from build123d import *

# Parameters (mm, degrees)
SKETCH1_R           = 2.1828125
BOSS_EXTRUDE1_DEPTH = 6.35
CHAMFER1_SIZE       = 0.396875


with BuildPart() as part:
    # Sketch1 → Boss-Extrude1 (new body)
    with BuildSketch(Plane(origin=(0, 0, 0), x_dir=(1, 0, 0), z_dir=(0, 1, 0))):
        with BuildLine():
            Line((-101.600254, 6.35), (0.000254, 6.35))
            ThreePointArc((0.000254, 6.35), (4.490202455, 4.490202455), (6.35, 0.000254))
            Line((6.35, 0.000254), (6.35, -12.700254))
            ThreePointArc((6.35, -12.700254), (4.490202455, -17.190202455), (0.000254, -19.05))
            ThreePointArc((0.000254, -19.05), (-4.490202455, -17.190202455), (-6.35, -12.700254))
            ThreePointArc((-6.35, -12.700254), (-8.209797545, -8.209797545), (-12.699746, -6.35))
            Line((-12.699746, -6.35), (-88.900254, -6.35))
            ThreePointArc((-88.900254, -6.35), (-93.390202455, -8.209797545), (-95.25, -12.699746))
            ThreePointArc((-95.25, -12.699746), (-97.109797545, -17.190202455), (-101.599746, -19.05))
            ThreePointArc((-101.599746, -19.05), (-106.090202455, -17.190202455), (-107.95, -12.700254))
            Line((-107.95, -12.700254), (-107.95, 0.000254))
            ThreePointArc((-107.95, 0.000254), (-106.090202455, 4.490202455), (-101.600254, 6.35))
        make_face()
        Circle(SKETCH1_R, mode=Mode.SUBTRACT)
        with Locations((-25.4, 0)):
            Circle(SKETCH1_R, mode=Mode.SUBTRACT)
        with Locations((-76.2, 0)):
            Circle(SKETCH1_R, mode=Mode.SUBTRACT)
        with Locations((-101.6, 0)):
            Circle(SKETCH1_R, mode=Mode.SUBTRACT)
        with Locations((-101.6, -12.7)):
            Circle(SKETCH1_R, mode=Mode.SUBTRACT)
        with Locations((0, -12.7)):
            Circle(SKETCH1_R, mode=Mode.SUBTRACT)
    extrude(amount=BOSS_EXTRUDE1_DEPTH)

    # Chamfer1
    chamfer1_edges = [part.edges().sort_by_distance(p)[0] for p in [
        (-4.490022844, 6.35, 17.19038206),
        (-50.8, 0, 6.35),
        (-93.390202455, 0, 8.209797545),
        (-97.10961794, 0, 17.190022844),
        (-4.490022844, 6.35, 17.19038206),
        (-97.10961794, 0, 17.190022844),
        (-106.090022844, 0, 17.19038206),
        (-106.090022844, 0, 17.19038206),
        (-107.95, 0, 6.35),
        (-106.090202455, 0, -4.490202455),
        (-50.8, 0, -6.35),
        (4.490202455, 0, -4.490202455),
        (6.35, 0, 6.35),
        (4.490202455, 0, 17.190202455),
        (-4.490022844, 0, 17.19038206),
        (4.490202455, 6.35, 17.190202455),
        (-4.490022844, 0, 17.19038206),
        (-8.20961794, 0, 8.209977156),
        (-8.20961794, 0, 8.209977156),
        (6.35, 6.35, 6.35),
        (4.490202455, 6.35, -4.490202455),
        (-50.8, 6.35, -6.35),
        (-106.090202455, 6.35, -4.490202455),
        (-2.1828125, 0, 0),
        (-2.1828125, 6.35, 0),
        (-107.95, 6.35, 6.35),
        (-27.5828125, 0, 0),
        (-27.5828125, 6.35, 0),
        (-106.090022844, 6.35, 17.19038206),
        (-78.3828125, 0, 0),
        (-78.3828125, 6.35, 0),
        (-106.090022844, 6.35, 17.19038206),
        (-8.20961794, 6.35, 8.209977156),
        (-103.7828125, 0, 0),
        (-103.7828125, 6.35, 0),
        (-97.10961794, 6.35, 17.190022844),
        (-103.7828125, 0, 12.7),
        (-103.7828125, 6.35, 12.7),
        (-97.10961794, 6.35, 17.190022844),
        (-2.1828125, 0, 12.7),
        (-2.1828125, 6.35, 12.7),
        (-93.390202455, 6.35, 8.209797545),
        (-50.8, 6.35, 6.35),
        (-8.20961794, 6.35, 8.209977156),
    ]]
    chamfer(chamfer1_edges, length=CHAMFER1_SIZE)


solid = part.part
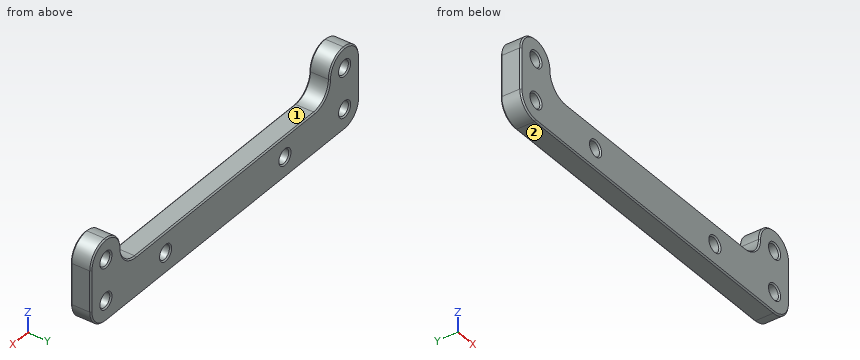
Part model, mm, in its own coordinate system. Face numbers are marked on the shaded views. A direction names the side the tool comes from. Coordinates: 2 decimals unless noted, no trailing zeros. Write each loop counter-clockwise with the first axis right and the second up, starting at its lowest first coordinate (ties: lowest second). Pieces come first, ordered by that corner, then holes. Notation, with made-up numbers: M 59.25,42 L 97.25,42 A29 cw 97.25,71 Z; hole C -13.5,69.5 d3. An arc over 180 degrees is marked long. Return JSON: item names as keys, results as strings.
1. Flat gauge pins, fed straight in: pin 1 Ø3 at (y, z) = (2.5, -3.5) entering from +X; pin 2 Ø5 at (x, z) = (-25.4, 0) entering from +Y; pin 3 Ø5 at (x, z) = (-93.5, 16) entering from +Y. Where does each tip first touch, or does it go through?
Determined:
{"pin 1": "x = 6.03", "pin 2": "y = 6.27", "pin 3": "y = 6.06"}
2. 3-axis set-ups, long thin cutter, end or side, ignore diameter. For the marked faces 1 and 2: which of +Z, -Z, +X, -X, +Y, -Y reach the whole face in a straight line?
Determined:
{"face 1": "+Z, +Y, -Y", "face 2": "-Z, +X, -X, +Y, -Y"}
3. Probe L1, parallel to Z at x = -101.6, y = 3.1; L2, parallel to Z at x = -25.4, y = 1.85; L3, parallel to X at y = 3.15, z = 0. List the from-to ranges inside material, lowest first.
Determined:
{"L1": "-6.35 to -2.18, 2.18 to 10.52, 14.88 to 19.05", "L2": "-6.35 to -2.18, 2.18 to 6.35", "L3": "-107.95 to -103.78, -99.42 to -78.38, -74.02 to -27.58, -23.22 to -2.18, 2.18 to 6.35"}
4. Saw through at C-C, the plane x = -45.5. Write the cut outline in (y, z), then the cut area to 3 significant figures.
Determined:
{"outline": "M 0,-5.95 L 0.4,-6.35 L 5.95,-6.35 L 6.35,-5.95 L 6.35,5.95 L 5.95,6.35 L 0.4,6.35 L 0,5.95 Z", "area": "80.3 mm²"}
5. Saw through at A-A, the plane y = 4.5. Write the cut outline in (x, z), then the cut area to 3 significant figures.
Determined:
{"outline": "M -107.95,0 A6.35 ccw -101.6,-6.35 L 0,-6.35 A6.35 ccw 6.35,0 L 6.35,12.7 A6.35 ccw 0,19.05 A6.35 ccw -6.35,12.7 A6.35 cw -12.7,6.35 L -88.9,6.35 A6.35 cw -95.25,12.7 A6.35 ccw -101.6,19.05 A6.35 ccw -107.95,12.7 Z; hole C -101.6,0 d4.37; hole C -101.6,12.7 d4.37; hole C -76.2,0 d4.37; hole C -25.4,0 d4.37; hole C 0,0 d4.37; hole C 0,12.7 d4.37", "area": "1,650 mm²"}
6. Saw through at B-B, the plane x = -76.2. Write the cut outline in (y, z), then the cut area to 3 significant figures.
Determined:
{"outline": "M 0,-5.95 L 0.4,-6.35 L 5.95,-6.35 L 6.35,-5.95 L 6.35,-2.58 L 5.95,-2.18 L 0.4,-2.18 L 0,-2.58 Z; M 0,2.58 L 0.4,2.18 L 5.95,2.18 L 6.35,2.58 L 6.35,5.95 L 5.95,6.35 L 0.4,6.35 L 0,5.95 Z", "area": "52.3 mm²"}
